Autodesk Inventor part; units mm, degrees
ref_plane "YZ Plane" through (0, 0, 0) normal (1, 0, 0) x (0, 1, 0)
ref_plane "XZ Plane" through (0, 0, 0) normal (0, 1, 0) x (-1, 0, 0)
ref_plane "XY Plane" through (0, 0, 0) normal (0, 0, 1) x (1, 0, 0)
sketch "Sketch1" plane through (0, 0, 0) normal (0, 0, 1) x (1, 0, 0)
  line L0 (14.5, -15) -> (-14.5, -15) construction
  line L1 (-14.5, -15) -> (-14.5, 15)
  line L2 (-14.5, 15) -> (14.5, 15)
  line L3 (14.5, 15) -> (14.5, -15)
  line L4 (14.5, -15) -> (-14.5, 15) construction
  line L5 (-14.5, -15) -> (14.5, 15) construction
  line L6 (-14.5, -15) -> (-18, -15)
  line L7 (-18, -15) -> (-18, 18.5)
  line L8 (-18, 18.5) -> (18, 18.5)
  line L9 (18, 18.5) -> (18, -15)
  line L10 (18, -15) -> (14.5, -15)
  point P0 (0, 0)
  dimension "d0" = 29
  dimension "d1" = 30
  dimension "d2" = 3.5
  dimension "d3" = 33.5
  dimension "d4" = 36
extrude "Extrusion1" add sketch "Sketch1" along normal blind 20
sketch "Sketch2" plane through (-18, -15, 0) normal (-1, 0, 0) x (0, 0, 1)
  arc A0 (0, 10) -> (20, 10) centre (10, 10) ccw
  line L0 (20, 33.5) -> (20, 0)
  line L1 (0, 0) -> (20, 0) construction
  line L2 (0, 10) -> (0, 0)
  line L3 (0, 0) -> (20, 0)
  line L4 (0, 0) -> (20, 0)
  line L5 (20, 0) -> (20, 10)
  circle A1 centre (10, 10) radius 3.4
  circle A2 centre (10, 10) radius 6 construction
  circle A3 centre (4, 10) radius 1
  circle A4 centre (16, 10) radius 1
  circle A5 centre (10, 16) radius 1
  circle A6 centre (10, 4) radius 1
  point P0 (0, 15)
  point P1 (10, 0)
  dimension "d7" = 20
  dimension "d8" = 10
  dimension "d9" = 10
  dimension "d10" = 6.8
  dimension "d11" = 12
  dimension "d12" = 2
  dimension "d13" = 2
  dimension "d14" = 2
  dimension "d15" = 2
extrude "Extrusion2" cut sketch "Sketch2" against normal through all
fillet "Fillet1" radius 5 4 edges at (-14.5, 15, 10) (14.5, 15, 10) (-18, 18.5, 10) (18, 18.5, 10)
sketch "Sketch3" plane through (-9.5, 15, 0) normal (0, -1, 0) x (1, 0, 0)
  line L0 (-8.2697, 20) -> (0, 20)
  line L1 (0, 20) -> (19, 20) construction
  line L2 (19, 20) -> (27.2697, 20)
  line L3 (27.2697, 20) -> (27.2697, 0)
  line L4 (27.2697, 0) -> (19, 0)
  line L5 (19, 20) -> (19, 0) construction
  line L6 (-8.2697, 0) -> (-8.2697, 20)
  line L7 (0, 0) -> (-8.2697, 0)
  line L8 (0, 20) -> (0, 0) construction
  line L9 (19, 0) -> (0, 0) construction
  line L10 (3.5, 16) -> (15.5, 16) construction
  line L11 (15.5, 16) -> (15.5, 4) construction
  line L12 (15.5, 4) -> (3.5, 4) construction
  line L13 (3.5, 4) -> (3.5, 16) construction
  line L14 (3.5, 16) -> (15.5, 4) construction
  line L15 (15.5, 16) -> (3.5, 4) construction
  circle A0 centre (3.5, 16) radius 1
  circle A1 centre (15.5, 16) radius 1
  circle A2 centre (3.5, 4) radius 1
  circle A3 centre (15.5, 4) radius 1
  point P0 (9.5, 0)
  point P1 (9.5, 10)
  dimension "d19" = 12
  dimension "d20" = 12
  dimension "d21" = 10
  dimension "d22" = 9.5
  dimension "d23" = 2
  dimension "d24" = 2
  dimension "d25" = 2
  dimension "d26" = 2
extrude "Extrusion3" cut sketch "Sketch3" against normal through all
sketch "Sketch4" plane through (-9.5, 15, 0) normal (0, -1, 0) x (1, 0, 0)
  circle A0 centre (3.5, 4) radius 1 construction
  circle A1 centre (15.5, 16) radius 1 construction
  circle A2 centre (15.5, 4) radius 1 construction
  circle A3 centre (3.5, 16) radius 1 construction
  line L0 (-8.2697, 20) -> (0, 20)
  line L1 (0, 20) -> (19, 20) construction
  line L2 (19, 20) -> (27.2697, 20)
  line L3 (27.2697, 20) -> (27.2697, 0)
  line L4 (27.2697, 0) -> (19, 0)
  line L5 (19, 20) -> (19, 0) construction
  line L6 (-8.2697, 0) -> (-8.2697, 20)
  line L7 (0, 0) -> (-8.2697, 0)
  line L8 (0, 20) -> (0, 0) construction
  line L9 (19, 0) -> (0, 0) construction
  circle A4 centre (3.5, 16) radius 2.25
  circle A5 centre (15.5, 16) radius 2.25
  circle A6 centre (15.5, 4) radius 2.25
  circle A7 centre (3.5, 4) radius 2.25
  point P0 (9.5, 0)
  dimension "d29" = 4.5
  dimension "d30" = 4.5
  dimension "d31" = 4.5
  dimension "d32" = 4.5
extrude "Extrusion4" cut sketch "Sketch4" against normal blind 1
properties part number "Motor_Bracket"
Input: part model. Units: mm. Frame: model coordinates. A direction names the side the tool comes from. Coordinates: 2 decimals unless noted, no trailing zeros. Write each loop counter-clockwise with the first axis right and the second up, starting at its lowest first coordinate (ties: lowest second). Pieces come first, ordered by that corner, then holes. Notation, with made-up numbers: M -7,-6 L 9,-6 A10 cw 9,9 Z; hole C -31.5,-6.5 d7. An arc over 180 degrees is marked long. Answer as a JSON object with one key per item and string values. Group by question number.
(1) Mould query, pull axis Y, two halves, no side actions, for faces 4 (the face through (-3.854, 15.493, 4.676)), 5 (the face through (0, 15, 10)), 6 (the face through (-16.274, -4.324, 3.263)). Classes: pulls with the +Y half, pulls with the -Y half, needs draft (parallel to the pull), parting line crosses it, or undercut.
(2) Contact query for flat-ended pins moving along their axis: P1, Ø2.5, axis at y = -5, z = 16, coming from the +X side; P2, Ø10, axis at x = -14.5, y = -11.5, coming from the +Z side; P3, Ø2.5, axis at x = 6, z = 16, coming from the -Y side; P4, Ø5, axis at x = 7, z = 3.5, coming from the -Y side. Output: stop coordinate, or through.
(3) Section A-A on y = -0.5. Output: boundary loops of the cut face in (x, z).
(4) Section B-B on x = -6. Output: boundary loops of the cut face in (y, z).
(5) Ray query, line 1 along Z through (x, y) = (6, 17.3); line 2 along X through (y, z) = (-9, 1.5); line 3 along Z through (x, y) = (-6, 15.5). Return the intervals inside material, ascending. Write a range as [from, to].
(6) Set-up query: faces 1 (the face through (7.038, 15.493, 14.004)), 2 (the face through (16, -5, 17)), 3 (the face through (14.5, -2, 8)). Return all of +Z, -Z, +X, -X, +Y, -Y with unobstructed straight access to the full face (end or side cutting, diameter ignored); none if empty.
(7) Section D-D on z = 12.5. Output: boundary loops of the cut face in (x, y), plus the area to 3 significant figures.
(8) Section C-C on y = -11. Output: boundary loops of the cut face in (x, z), plus the area to 3 significant figures.
Result set:
{
 "1": {"face 4": "needs draft", "face 5": "pulls with the -Y half", "face 6": "undercut"},
 "2": {"P1": "stops at x = 18", "P2": "stops at z = 19.89", "P3": "stops at y = 16", "P4": "stops at y = 15"},
 "3": {"outline": "M -18,0 L -14.5,0 L -14.5,20 L -18,20 Z; M 14.5,0 L 18,0 L 18,20 L 14.5,20 Z"},
 "4": {"outline": "M 15,0 L 18.5,0 L 18.5,3 L 16,3 L 16,1.75 L 15,1.75 Z; M 15,6.25 L 16,6.25 L 16,5 L 18.5,5 L 18.5,15 L 16,15 L 16,13.75 L 15,13.75 Z; M 15,18.25 L 16,18.25 L 16,17 L 18.5,17 L 18.5,20 L 15,20 Z"},
 "5": {"line 1": "z = [0, 3], [5, 15], [17, 20]", "line 2": "x = [-18, -14.5], [14.5, 18]", "line 3": "z = [0, 1.75], [6.25, 13.75], [18.25, 20]"},
 "6": {"face 1": "-Y", "face 2": "+X, -X", "face 3": "+Z, -Z, -Y"},
 "7": {"outline": "M -18,-14.68 L -14.5,-14.68 L -14.5,-7.3 L -18,-7.3 Z; M -18,-2.7 L -14.5,-2.7 L -14.5,10 A5 cw -9.5,15 L 9.5,15 A5 cw 14.5,10 L 14.5,-2.7 L 18,-2.7 L 18,13.5 A5 ccw 13,18.5 L -13,18.5 A5 ccw -18,13.5 Z; M 14.5,-14.68 L 18,-14.68 L 18,-7.3 L 14.5,-7.3 Z", "area": "302 mm2"},
 "8": {"outline": "M -18,2 L -14.5,2 L -14.5,9 L -18,9 Z; M -18,11 L -14.5,11 L -14.5,18 L -18,18 Z; M 14.5,2 L 18,2 L 18,9 L 14.5,9 Z; M 14.5,11 L 18,11 L 18,18 L 14.5,18 Z", "area": "98.0 mm2"}
}
